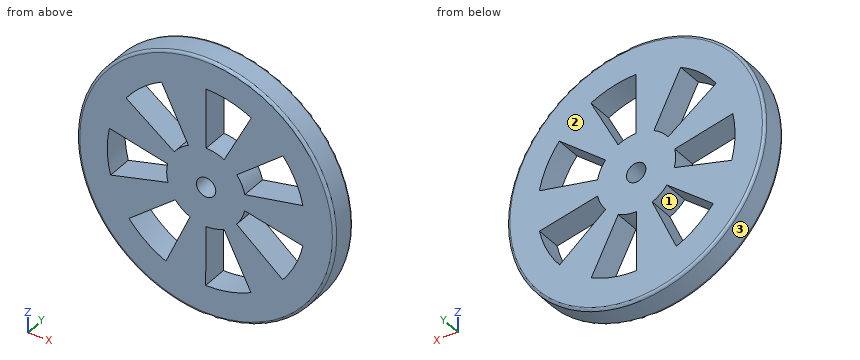
```python
from build123d import *

# Parameters (mm, degrees)
SKETCH1_R           = 100
BOSS_EXTRUDE1_DEPTH = 20
FILLET1_R           = 2
SKETCH2_R           = 7.5
CUT_EXTRUDE1_DEPTH  = 21
CUT_EXTRUDE2_DEPTH  = 21
CIRPATTERN1_COUNT   = 7
CIRPATTERN1_ANGLE   = 306


with BuildPart() as part:
    # Sketch1 → Boss-Extrude1 (new body)
    with BuildSketch(Plane(origin=(0, 0, 0), x_dir=(1, 0, 0), z_dir=(0, 1, 0))):
        Circle(SKETCH1_R)
    extrude(amount=BOSS_EXTRUDE1_DEPTH)

    # Fillet1
    fillet1_edges = [part.edges().sort_by_distance(p)[0] for p in [
        (-100, 0, 0),
        (-100, 20, 0),
    ]]
    fillet(fillet1_edges, radius=FILLET1_R)

    # Sketch2 → Cut-Extrude1 (cut, through all)
    with BuildSketch(Plane(origin=(0, 20, 0), x_dir=(1, 0, 0), z_dir=(0, 1, 0))):
        Circle(SKETCH2_R)
    extrude(amount=-CUT_EXTRUDE1_DEPTH, mode=Mode.SUBTRACT)

    # Sketch3 → Cut-Extrude2 (cut, through all)
    with BuildSketch(Plane.XZ):
        with BuildLine():
            Line((0, 30.617728898), (0, 76.732128088))
            ThreePointArc((0, 76.732128088), (18.073615255, 74.573211762), (35.130200903, 68.217948265))
            Line((35.130200903, 68.217948265), (14.017687169, 27.220392527))
            ThreePointArc((14.017687169, 27.220392527), (7.21175166, 29.756275991), (0, 30.617728898))
        make_face()
    cut_extrude2 = extrude(amount=-CUT_EXTRUDE2_DEPTH, mode=Mode.SUBTRACT)

    # CirPattern1: Cut-Extrude2 ×7 about axis
    cirpattern1_axis = Axis((0, 0, 0), (0, 1, 0))
    for i in range(1, CIRPATTERN1_COUNT):
        add(cut_extrude2.rotate(cirpattern1_axis, i * CIRPATTERN1_ANGLE / (CIRPATTERN1_COUNT - 1)), mode=Mode.SUBTRACT)


solid = part.part
```
The listing builds one solid part. Answer for the finished solid, in the listing's coordinates (mm). Face numbers are marked on the shaded views. Round coordinates to 2 decimals unless told otherwise and drop trailing zeros. Order: outer loops, then holes, each group sorted by start corner. A loop starts at its lowest first (then second) coordinate and runs counter-clockwise, first axis right, second up. Notation, with made-up numbers: (-40, 83) - (8, 83) arc R21 cw to (8, 91) - close; hole circle Ø5 at (-25, 63.25). An arc over 180 degrees is marked (long way). Put each result on its own line as item: value. Start each with the question number.
(1) Determine the mould class of the marked faces 1, 2 and 3 for opening direction X: released by +X, released by -X, zero draft, split by the parting line, or undercut.
(2) Given P1, Ø8, axis at y = 9, z = -71.5, coming from the -X side; P2, Ø6, axis at y = 7, z = -31, coming from the +X side; P3, Ø6, axis at x = -34.5, y = 2.5, coming from the -Z side, each flat-ended and moving along its own axis, determine where each tip first touches the part or whether it passes through.
(3) Straight lines are drawn through the part: probe 1 along X at (y, z) = (16.25, 0); probe 2 along X at (y, z) = (5.5, -60); probe 3 along Z at (x, y) = (-44, 17.25). For each, find the intervals that lie inside material, in ascending order. Write a range as from..to.
(4) Find section B-B (z = 0). Give the vertices of the cut face in (x, y).
(5) Find section A-A (y = 5.75). State how many separate pieces and enclosed holes the cut face has, plus the area to 3 significant figures.
Reply:
1. face 1: undercut
1. face 2: zero draft
1. face 3: split by the parting line
2. P1: x = -73.78
2. P2: x = 96
2. P3: z = -94.91
3. probe 1: -100..-76.73, -30.62..-7.5, 7.5..100
3. probe 2: -80..-47.83, -26.71..-0.26, 30.57..80
3. probe 3: -89.8..-62.86, -35.32..-11.79, 9.55..31.97, 62.86..89.8
4. outline: (-100, 2) arc R2 ccw to (-98, 0) - (-76.73, 0) - (-76.73, 20) - (-98, 20) arc R2 ccw to (-100, 18) - close; (-30.62, 0) - (-7.5, 0) - (-7.5, 20) - (-30.62, 20) - close; (7.5, 0) - (98, 0) arc R2 ccw to (100, 2) - (100, 18) arc R2 ccw to (98, 20) - (7.5, 20) - close
5. separate pieces: 1
5. enclosed holes: 8
5. area: 23,000 mm^2
